```python
from build123d import *

# Parameters (mm, degrees)
SKETCH1_W           = 50
SKETCH1_H           = 35
BOSS_EXTRUDE1_DEPTH = 4.6
SKETCH2_W           = 22.6
SKETCH2_H           = 11.6
CUT_EXTRUDE1_DEPTH  = 62.20588207
SKETCH3_R           = 3
BOSS_EXTRUDE2_DEPTH = 4.4
SKETCH5_W           = 50
SKETCH5_H           = 2.5
BOSS_EXTRUDE3_DEPTH = 4.6
SKETCH6_R           = 1.6
CUT_EXTRUDE2_DEPTH  = 64.144675152
SKETCH7_W           = 50
SKETCH7_H           = 1.5
BOSS_EXTRUDE4_DEPTH = 4.6
SKETCH8_W           = 1.45
SKETCH8_H           = 39
BOSS_EXTRUDE5_DEPTH = 4.6
SKETCH9_W           = 40
SKETCH9_H           = 5
BOSS_EXTRUDE6_DEPTH = 20.4
SKETCH10_R          = 2.1
CUT_EXTRUDE3_DEPTH  = 69.161572752
SKETCH11_R          = 1.1
CUT_EXTRUDE4_DEPTH  = 66.745037836
SKETCH12_W          = 2
SKETCH12_H          = 39
BOSS_EXTRUDE7_DEPTH = 4.6
CUT_EXTRUDE5_DEPTH  = 68.278599867
FILLET1_R           = 2
FILLET2_R           = 2


with BuildPart() as part:
    # Sketch1 → Boss-Extrude1 (new body)
    with BuildSketch(Plane(origin=(0, 0, 0), x_dir=(1, 0, 0), z_dir=(0, 1, 0))):
        with Locations((25, -17.5)):
            Rectangle(SKETCH1_W, SKETCH1_H)
    extrude(amount=BOSS_EXTRUDE1_DEPTH)

    # Sketch2 → Cut-Extrude1 (cut, through all)
    with BuildSketch(Plane(origin=(0, 4.6, 0), x_dir=(1, 0, 0), z_dir=(0, 1, 0))):
        with Locations((33.7, -17.5)):
            Rectangle(SKETCH2_W, SKETCH2_H)
    extrude(amount=-CUT_EXTRUDE1_DEPTH, mode=Mode.SUBTRACT)

    # Sketch3 → Boss-Extrude2 (add)
    with BuildSketch(Plane(origin=(0, 4.6, 0), x_dir=(1, 0, 0), z_dir=(0, 1, 0))):
        with Locations(Location((8.55, -17.5, 0), (0, 0, 270))):
            Circle(SKETCH3_R)
        with Locations(Location((15.54, -32.5, 0), (0, 0, 303.557309762))):
            Circle(SKETCH3_R)
        with Locations(Location((21.56, -32.5, 0), (0, 0, 303.557309762))):
            Circle(SKETCH3_R)
    extrude(amount=BOSS_EXTRUDE2_DEPTH)

    # Sketch5 → Boss-Extrude3 (add)
    with BuildSketch(Plane(origin=(0, 4.6, 0), x_dir=(1, 0, 0), z_dir=(0, 1, 0))):
        with Locations((25, -36.25)):
            Rectangle(SKETCH5_W, SKETCH5_H)
    extrude(amount=-BOSS_EXTRUDE3_DEPTH)

    # Sketch6 → Cut-Extrude2 (cut, through all)
    with BuildSketch(Plane(origin=(0, 9, 0), x_dir=(1, 0, 0), z_dir=(0, 1, 0))):
        with Locations(Location((8.55, -17.5, 0), (0, 0, 270))):
            Circle(SKETCH6_R)
        with Locations(Location((15.54, -32.5, 0), (0, 0, 270))):
            Circle(SKETCH6_R)
        with Locations(Location((21.56, -32.5, 0), (0, 0, 270))):
            Circle(SKETCH6_R)
    extrude(amount=-CUT_EXTRUDE2_DEPTH, mode=Mode.SUBTRACT)

    # Sketch7 → Boss-Extrude4 (add)
    with BuildSketch(Plane(origin=(0, 4.6, 0), x_dir=(1, 0, 0), z_dir=(0, 1, 0))):
        with Locations((25, 0.75)):
            Rectangle(SKETCH7_W, SKETCH7_H)
    extrude(amount=-BOSS_EXTRUDE4_DEPTH)

    # Sketch8 → Boss-Extrude5 (add)
    with BuildSketch(Plane(origin=(0, 4.6, 0), x_dir=(1, 0, 0), z_dir=(0, 1, 0))):
        with Locations((-0.725, -18)):
            Rectangle(SKETCH8_W, SKETCH8_H)
    extrude(amount=-BOSS_EXTRUDE5_DEPTH)

    # Sketch9 → Boss-Extrude6 (add)
    with BuildSketch(Plane(origin=(0, 4.6, 0), x_dir=(1, 0, 0), z_dir=(0, 1, 0))):
        with Locations((18.55, -1)):
            Rectangle(SKETCH9_W, SKETCH9_H)
    extrude(amount=BOSS_EXTRUDE6_DEPTH)

    # Sketch10 → Cut-Extrude3 (cut, through all)
    with BuildSketch(Plane(origin=(0, 0, -1.5), x_dir=(-1, 0, 0), z_dir=(0, 0, -1))):
        with Locations((-29.55, 15)):
            Circle(SKETCH10_R)
        with Locations((-7.55, 15)):
            Circle(SKETCH10_R)
    extrude(amount=-CUT_EXTRUDE3_DEPTH, mode=Mode.SUBTRACT)

    # Sketch11 → Cut-Extrude4 (cut, through all)
    with BuildSketch(Plane(origin=(0, 4.6, 0), x_dir=(1, 0, 0), z_dir=(0, 1, 0))):
        with Locations(Location((47.65, -17.5, 0), (0, 0, 270))):
            Circle(SKETCH11_R)
        with Locations(Location((19.75, -17.5, 0), (0, 0, 270))):
            Circle(SKETCH11_R)
    extrude(amount=-CUT_EXTRUDE4_DEPTH, mode=Mode.SUBTRACT)

    # Sketch12 → Boss-Extrude7 (add)
    with BuildSketch(Plane(origin=(0, 4.6, 0), x_dir=(1, 0, 0), z_dir=(0, 1, 0))):
        with Locations((51, -18)):
            Rectangle(SKETCH12_W, SKETCH12_H)
    extrude(amount=-BOSS_EXTRUDE7_DEPTH)

    # Sketch13 → Cut-Extrude5 (cut, through all)
    with BuildSketch(Plane(origin=(0, 4.6, 0), x_dir=(1, 0, 0), z_dir=(0, 1, 0))):
        Polygon((10.54, -37.5), (-1.45, -27.5), (-1.45, -37.5), align=None)
        Polygon((26.56, -37.5), (38.549602016, -27.5), (52, -27.5), (52, -37.5), align=None)
    extrude(amount=-CUT_EXTRUDE5_DEPTH, mode=Mode.SUBTRACT)

    # Fillet1
    fillet1_edges = [part.edges().sort_by_distance(p)[0] for p in [
        (52, 2.3, -1.5),
        (10.54, 2.3, 37.5),
        (-1.45, 2.3, 27.5),
        (26.56, 2.3, 37.5),
        (38.549602016, 2.3, 27.5),
        (52, 2.3, 27.5),
    ]]
    fillet(fillet1_edges, radius=FILLET1_R)

    # Fillet2
    fillet2_edges = [part.edges().sort_by_distance(p)[0] for p in [
        (-1.45, 25, 1),
        (38.55, 25, 1),
    ]]
    fillet(fillet2_edges, radius=FILLET2_R)


solid = part.part
```
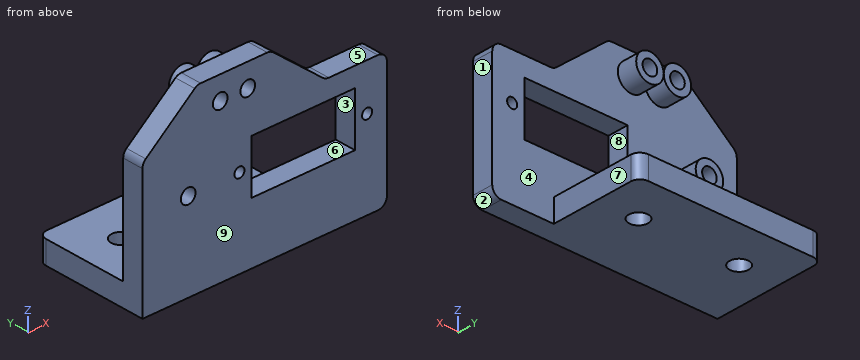
For this review, take the finished solid that the model builds, in its own axes (mm). Face numbers are marked on the shaded views. A direction names the side the tool comes from. Round coordinates to 2 decimals unless told otherwise and drop trailing zeros. Write each loop counter-clockwise with the first axis right and the second up, starting at its lowest first coordinate (ties: lowest second). Pieces come first, ordered by that corner, then holes. Notation, with made-up numbers: (-14.75, -21) - (12.25, -21) arc R22 cw to (12.25, -12) - close; hole circle Ø3 at (-27.75, -27.75). An arc over 180 degrees is marked (long way). Write each question's results on one line, items separated by ' | '.
Item 1: For the marked faces 1, 2, 3, 4 and 5, list the 3-axis set-ups (+Z, -Z, +X, -X, +Y, -Y) from which the entire face can be reached by the end or side of a thin tool; tool diameter is ignored.
Calculated:
face 1: +Z, -Z, +X, +Y, -Y | face 2: -Z, +X, +Y, -Y | face 3: +Y, -Y | face 4: +Y | face 5: +Z, +X, +Y, -Y
Item 2: For pin 1 (1.5 mm diameter, centred on y = 10, z = 22.5, fed in from +X); pin 2 (4 mm diameter, centred on y = 14.5, z = 2, fed in from +X); pin 3 (10 mm diameter, centred on x = 22, y = 10.5, fed in from +Z); pin 4 (2.5 mm diameter, centred on x = 30, y = 3, fed in from +Z), all flat-tipped, find the tip position at first contact; note any pin that passes through.
Calculated:
pin 1: passes through | pin 2: stops at x = 38.55 | pin 3: stops at z = 35.5 | pin 4: stops at z = 35.67
Item 3: Take a section at D-D on x = 8.55. State the section outline as (y, z) points.
Calculated:
outline: (0, -1.5) - (13.15, -1.5) - (13.15, 3.5) - (4.6, 3.5) - (4.6, 14.5) - (9, 14.5) - (9, 15.9) - (0, 15.9) - close; (0, 19.1) - (9, 19.1) - (9, 20.5) - (4.6, 20.5) - (4.6, 35.84) - (0, 35.84) - close; (16.85, -1.5) - (25, -1.5) - (25, 3.5) - (16.85, 3.5) - close
Item 4: Take a section at A-A on x = 47.65. State the section outline as (y, z) points.
Calculated:
outline: (0, -1.5) - (4.6, -1.5) - (4.6, 16.4) - (0, 16.4) - close; (0, 18.6) - (4.6, 18.6) - (4.6, 27.5) - (0, 27.5) - close
Item 5: Take a section at B-B on y = 3.5. State the section outline as (x, z) points, then the cut area to 3 significant figures.
Calculated:
outline: (-1.45, -1.5) - (50, -1.5) arc R2 ccw to (52, 0.5) - (52, 25.5) arc R2 ccw to (50, 27.5) - (39.27, 27.5) arc R2 cw to (37.99, 27.96) - (27.12, 37.04) arc R2 ccw to (25.84, 37.5) - (11.26, 37.5) arc R2 ccw to (9.98, 37.04) - (-0.73, 28.1) arc R2 ccw to (-1.45, 26.56) - close; hole circle Ø3.2 at (8.55, 17.5); hole circle Ø3.2 at (15.54, 32.5); hole circle Ø2.2 at (19.75, 17.5); hole circle Ø3.2 at (21.56, 32.5); hole (22.4, 11.7) - (45, 11.7) - (45, 23.3) - (22.4, 23.3) - close; hole circle Ø2.2 at (47.65, 17.5) | area: 1,530 mm^2
Item 6: To check wall thickness, follow line 1 along X through (y, z) = (4, 17.5); line 2 along X through (y, z) = (4.75, 17.5); line 3 along X through (y, z) = (4.5, 32.5) (3 decimals). State the ranges of each line that lie inside material, in increasing order. Write a range as from..to.
Calculated:
line 1: x = -1.45..6.95, 10.15..18.65, 20.85..22.4, 45..46.55, 48.75..52 | line 2: x = 5.55..6.95, 10.15..11.55 | line 3: x = 4.545..13.94, 17.14..19.96, 23.16..32.555
Item 7: Take a section at C-C on z = 17.5. State the section outline as (x, y) points, then the cut area to 3 significant figures.
Calculated:
outline: (-1.45, 0) - (6.95, 0) - (6.95, 9) - (5.55, 9) - (5.55, 4.6) - (-1.45, 4.6) - close; (10.15, 0) - (18.65, 0) - (18.65, 4.6) - (11.55, 4.6) - (11.55, 9) - (10.15, 9) - close; (20.85, 0) - (22.4, 0) - (22.4, 4.6) - (20.85, 4.6) - close; (45, 0) - (46.55, 0) - (46.55, 4.6) - (45, 4.6) - close; (48.75, 0) - (52, 0) - (52, 4.6) - (48.75, 4.6) - close | area: 119 mm^2
Item 8: Draft analysis for pull direction X (two halves, no side actions). For the marked faces 6, 7, 8 and 9, state which applies: pulls with the +X half, pulls with the -X half, needs draft (parallel to the pull), parting line crosses it, or undercut.
Calculated:
face 6: undercut | face 7: pulls with the +X half | face 8: undercut | face 9: needs draft
